Geometry: see drawing. Coordinates: mm, zero at the bounding-box minimum. A direction names the side the tool comes from. Give positions to 0.01 mm unless a question says otherwise; leave off trailing zeros. Write each loop counter-clockwise with the first axis right and the second up, starting at its lowest first coordinate (ties: lowest second). Pieces come first, ordered by that corner, then holes. Notation, with made-up numbers: (30, 50) - (60, 50) arc R23 ccw to (60, 59) - close; hole circle Ø6 at (19, -36.75). An arc over 180 degrees is marked (long way). Use a Markdown table: item, result. Add a question column.
1. Section query C-C, the plane x = 18. Return loops of the section in (y, z).
2. Section query D-D, the plane x = 24. Return loops of the section in (y, z), plus the area to 3 significant figures.
3. Material intervals for probe 1 along X at (y, z) = (1.5, 1.25); probe 2 along Y at (x, z) = (31, 4.25); probe 3 along X at (y, z) = (2.75, 3.75), sorted ascending.
4. Mould query, pull axis Y, two halves, no side actions, for the marked faces 1, 2 and 3. Classes: released by +Y, released by -Y, zero draft, split by the parting line, or undercut.
5. Section query A-A, the plane y = 4. Return loops of the section in (x, z), plus the area to 3 significant figures.
6. Set-up query: the marked faces 4 and 5. Return all of +Z, -Z, +X, -X, +Y, -Y with unobstructed straight access to the full face (end or side cutting, diameter ignored); none if empty.
7. Section query B-B, the plane z = 4. Return loops of the section in (x, y), plus the area to 3 significant figures.
8. Pin query (flat end, axial travel): pin 1 (4 mm diameter, centred on x = 19.5, z = 1.5, fed in from +Y); pin 2 (1 mm diameter, centred on y = 6, z = 6.5, fed in from +X); pin 3 (2 mm diameter, centred on y = 3, z = 1.5, fed in from -X). Return the tip coordinate at first contact, or that it passes through.
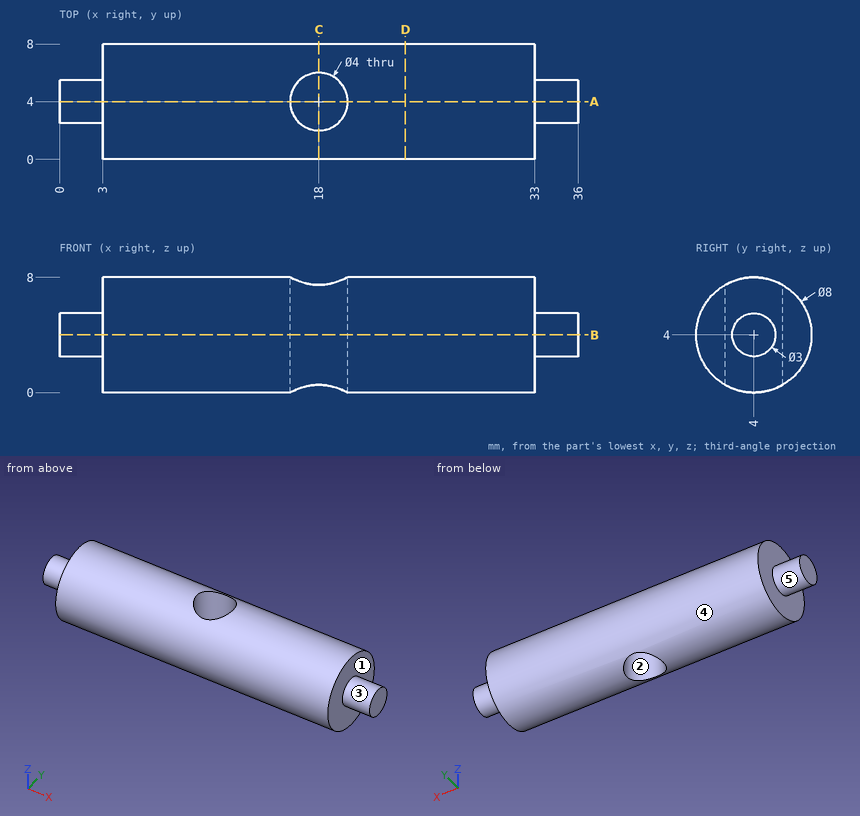
Result sheet:
| question | item | result |
|---|---|---|
| 1 | outline | (2, 0.54) - (2, 7.46) arc R4 ccw to start; (6, 0.54) arc R4 ccw to (6, 7.46) - close |
| 2 | outline | circle Ø8 at (4, 4) |
| 2 | area | 50.3 mm² |
| 3 | probe 1 | x = 3 to 33 |
| 3 | probe 2 | y = 0.01 to 7.99 |
| 3 | probe 3 | x = 0 to 16.44, 19.56 to 36 |
| 4 | face 1 | zero draft |
| 4 | face 2 | undercut |
| 4 | face 3 | split by the parting line |
| 5 | outline | (0, 2.5) - (3, 2.5) - (3, 0) - (16, 0) - (16, 8) - (3, 8) - (3, 5.5) - (0, 5.5) - close; (20, 0) - (33, 0) - (33, 2.5) - (36, 2.5) - (36, 5.5) - (33, 5.5) - (33, 8) - (20, 8) - close |
| 5 | area | 226 mm² |
| 6 | face 4 | +X, -X |
| 6 | face 5 | -X |
| 7 | outline | (0, 2.5) - (3, 2.5) - (3, 0) - (33, 0) - (33, 2.5) - (36, 2.5) - (36, 5.5) - (33, 5.5) - (33, 8) - (3, 8) - (3, 5.5) - (0, 5.5) - close; hole circle Ø4 at (18, 4) |
| 7 | area | 245 mm² |
| 8 | pin 1 | stops at y = 7.97 |
| 8 | pin 2 | stops at x = 33 |
| 8 | pin 3 | stops at x = 3 |
